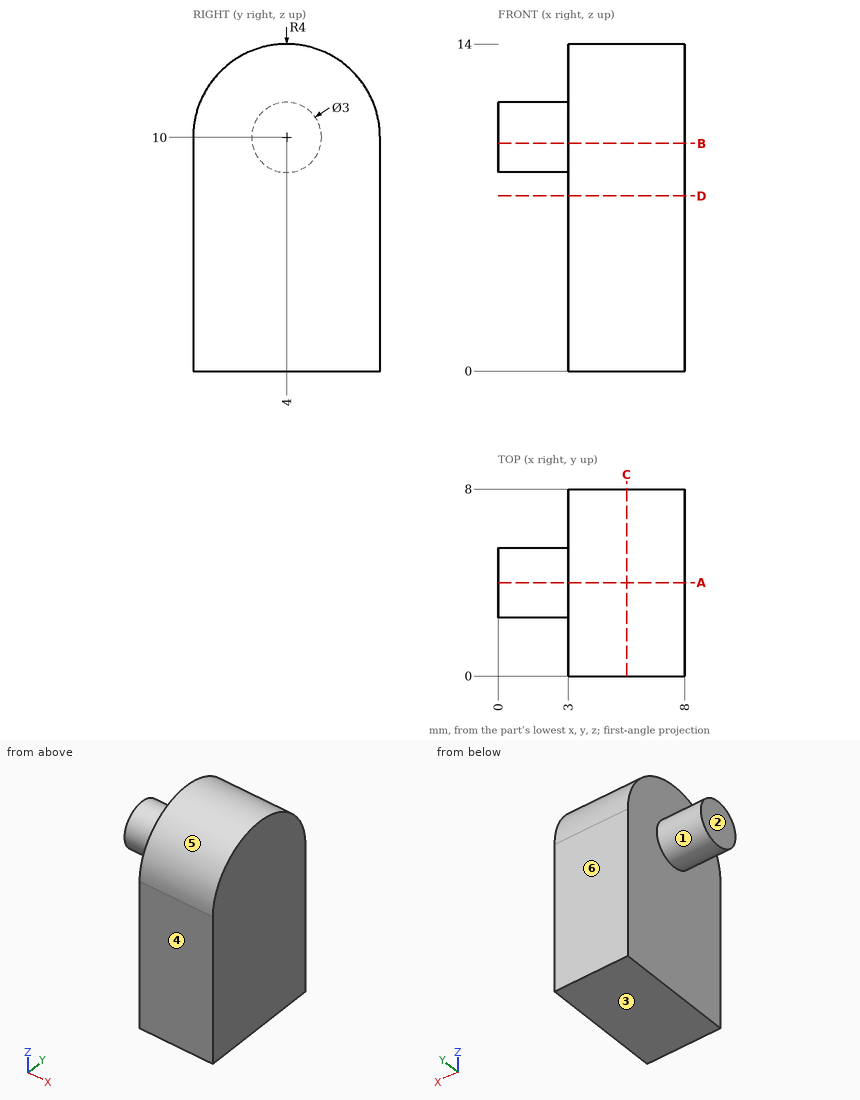
Job drawing, mm, ordinate dimensions from the low corner. One solid piece. A direction names the side the tool comes from. Round coordinates to 2 decimals unless told otherwise and drop trailing zeros. Loops run counter-clockwise (first coordinate to the right, second up) from the corner with the lowest first, then second, coordinate; pieces in that order, holes last.
(1) Cut at A-A (y = 4). Give the cut face in (x, z), plus the area to 3 significant figures.
(2) Two-plate mould, pull along Y, no slides. Class the marked faces 3, 4, 5 and 6: +Y half, -Y half, draft (parallel to the pull), parting line (faces both ways), or undercut.
(3) Wall check: line 1 along X through (y, z) = (2.75, 7); line 2 along Z through (x, y) = (7.75, 1.25); line 3 along Z through (x, y) = (7.75, 2.5). Give the ranges that are in metal, low to high.
(4) Cut at C-C (x = 5.5). Give the cut face in (y, z), plus the area to 3 significant figures.
(5) Cut at B-B (z = 9.75). Give the cut face in (x, y), plus the area to 3 significant figures.
(6) Cut at D-D (z = 7.5). Give the cut face in (x, y).
(7) Drop flat-ended pins along their axis: pin 1 (2 mm diameter, centred on x = 6.5, z = 9.5, fed in from -Y); pin 2 (3 mm diameter, centred on x = 4.5, y = 1.5, fed in from +Z). Give the stop position or say it passes through.
(8) Which spindle directions (+Z, -Z, +X, -X, +Y, -Y) get a long thin tool onto all of the face, cutting with end or side? Do the marked faces 1 and 2. Say none if no direction does.
Findings below:
1. outline: (0, 8.5) - (3, 8.5) - (3, 0) - (8, 0) - (8, 14) - (3, 14) - (3, 11.5) - (0, 11.5) - close
1. area: 79.0 mm2
2. face 3: draft
2. face 4: -Y half
2. face 5: parting line
2. face 6: +Y half
3. line 1: x = 3 to 8
3. line 2: z = 0 to 12.9
3. line 3: z = 0 to 13.71
4. outline: (0, 0) - (8, 0) - (8, 10) arc R4 ccw to (0, 10) - close
4. area: 105 mm2
5. outline: (0, 2.52) - (3, 2.52) - (3, 0) - (8, 0) - (8, 8) - (3, 8) - (3, 5.48) - (0, 5.48) - close
5. area: 48.9 mm2
6. outline: (3, 0) - (8, 0) - (8, 8) - (3, 8) - close
7. pin 1: stops at y = 0
7. pin 2: stops at z = 13.87
8. face 1: -X
8. face 2: +Z, -Z, -X, +Y, -Y
